For this review, take the finished solid that the model builds, in its own axes (mm). Coordinates: 2 decimals unless noted, no trailing zeros. Loops run counter-clockwise (first coordinate to the right, second up) from the corner with the lowest first, then second, coordinate; pieces in that order, holes last. Notation, with made-up numbers: M -26,-8 L -4,-8 A14 cw -4,2 Z; hole C 73.5,50 d8. An arc over 180 degrees is marked long. Use one line per item in the form item = value.
```python
from build123d import *

# Parameters (mm, degrees)
EXTRUDE_1_DEPTH          = 4
CUT_EXTRUDE_1_DEPTH      = 72.212602073
CUT_EXTRUDE_1_DEPTH_BACK = 72.212602073
SKETCH_7_R               = 1.5


with BuildPart() as part:
    # 草图1 → 凸台-拉伸1 (new body)
    with BuildSketch(Plane.XY):
        Polygon((-42.136394103, 0), (41.863605897, 0), (41.863605897, 57.269180071), (33.918605897, 57.269180071), (33.918605897, 32.269180071), (12.363605897, 32.269180071), (12.363605897, 57.269180071), (-12.636394103, 57.269180071), (-12.636394103, 32.269180071), (-34.191394103, 32.269180071), (-34.191394103, 57.269180071), (-42.136394103, 57.269180071), align=None)
    extrude(amount=EXTRUDE_1_DEPTH)

    # 草图7 → 切除-拉伸1 (cut, two sides: drawn at the far end of the back side and taken through both)
    with BuildSketch(Plane.XY.offset(4).offset(-CUT_EXTRUDE_1_DEPTH_BACK)):
        with Locations((-38.253699842, 4.077877428)):
            Circle(SKETCH_7_R)
        with Locations((-38.253699842, 35.306046983)):
            Circle(SKETCH_7_R)
        with Locations(Location((37.980911635, 35.306046983, 0), (0, 0, 180))):
            Circle(SKETCH_7_R)
        with Locations(Location((37.980911635, 4.077877428, 0), (0, 0, 180))):
            Circle(SKETCH_7_R)
    extrude(amount=CUT_EXTRUDE_1_DEPTH + CUT_EXTRUDE_1_DEPTH_BACK, mode=Mode.SUBTRACT)


solid = part.part
```
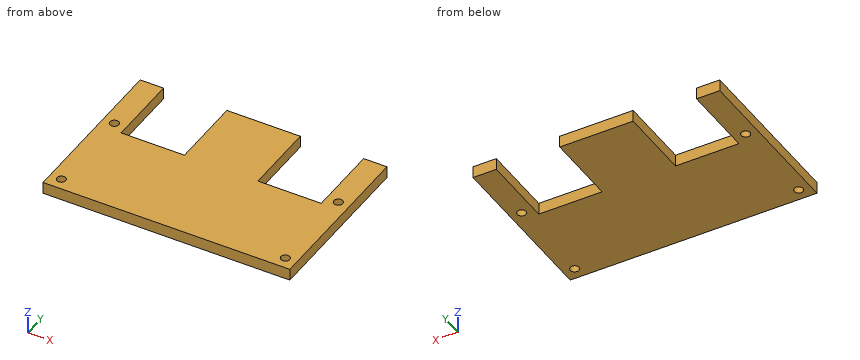
1. For pin 1 Ø2 at (x, z) = (-22.5, 2) entering from +Y, flat-tipped, find the tip position at first contact; note if it passes through.
Computed values:
pin_1 = 32.27
2. Consider section B-B on z = 1.4. Write out the cut boundary in (x, y), plus the area to 3 significant figures.
Computed values:
outline = M -42.14,0 L 41.86,0 L 41.86,57.27 L 33.92,57.27 L 33.92,32.27 L 12.36,32.27 L 12.36,57.27 L -12.64,57.27 L -12.64,32.27 L -34.19,32.27 L -34.19,57.27 L -42.14,57.27 Z; hole C -38.25,4.08 d3; hole C -38.25,35.31 d3; hole C 37.98,4.08 d3; hole C 37.98,35.31 d3
area = 3,700 mm2
3. Consider section C-C on x = 20. Write out the cut boundary in (y, z).
Computed values:
outline = M 0,0 L 32.27,0 L 32.27,4 L 0,4 Z
4. Consider section A-A on y = 38. Write out the cut boundary in (x, z).
Computed values:
outline = M -42.14,0 L -34.19,0 L -34.19,4 L -42.14,4 Z; M -12.64,0 L 12.36,0 L 12.36,4 L -12.64,4 Z; M 33.92,0 L 41.86,0 L 41.86,4 L 33.92,4 Z
5. Wall thickness on line 1 along X through (y, z) = (4, 1.3); line 2 along X through (y, z) = (44.5, 2.8); line 3 along X through (y, z) = (35.5, 0.5): over which ranges is each line inside the solid? List them lowest first. Write a range as from..to.
Computed values:
line_1 = -42.14..-39.75, -36.76..36.48, 39.48..41.86
line_2 = -42.14..-34.19, -12.64..12.36, 33.92..41.86
line_3 = -42.14..-39.74, -36.77..-34.19, -12.64..12.36, 33.92..36.49, 39.47..41.86
